CAD build for the part. Positions are in the model's coordinates, mm. A direction names the side the tool comes from. Coordinates: 2 decimals unless noted, no trailing zeros. Write each loop counter-clockwise with the first axis right and the second up, starting at its lowest first coordinate (ties: lowest second). Pieces come first, ordered by that corner, then holes. Notation, with made-up numbers: (-1.5, -24) - (11.5, -24) arc R13 ccw to (11.5, 1) - close; hole circle Ø8 at (52, -38). An arc over 180 degrees is marked (long way). Answer in a Markdown table with one row per item. Add a question column.
Q1. Band-saw the part on D-D (z = 19). List the corners of the cut face in (x, y), and give its area (3 significant figures).
Q2. 3-axis set-ups, long thin cutter, end or side, ignore diameter. For faces 4 (the flat face through (67.5, 25, 17)), 5 (the flat face through (16, 10, 17)), 6 (the flat face through (38, 40, 17)), 7 (the flat face through (72.5, 23, 21)): which of +Z, -Z, +X, -X, +Y, -Y reach the whole face in a straight line?
Q3. Drill centre lines: line 1 along Y through (x, z) = (62, 22); line 2 along X through (y, z) = (21, 26); line 3 along Y through (x, z) = (34.5, 25). Where is each one in solid material? Low to high. Write a range as from..to.
Q4. Band-saw the part on B-B (x = 61). List the corners of the cut face in (y, z).
Q5. Two-plate mould, pull along Y, no slides. Class faces 1 (the flat face through (75, 25, 2)), 2 (the cylindrical face through (1, 48, 3)), 3 (the flat face through (19, 15, 17)): +Y half, -Y half, draft (parallel to the pull), parting line (faces both ways), or undercut.
Q6. Band-saw the part on C-C (y = 25.5). List the corners of the cut face in (x, z), and give its area (3 significant figures).
Q7. Pin check, flat tips, straight feed: pin 1 (1 mm diameter, centred on x = 56, z = 26.5, fed in from -Y); pin 2 (20 mm diameter, centred on x = 29, y = 28, fed in from +Z); pin 3 (7 mm diameter, centred on x = 16, z = 17, fed in from +Y). Stop position of each tip, or through.
Q8. Band-saw the part on A-A (x = 35.5). List the corners of the cut face in (y, z), and give its area (3 significant figures).
```python
from build123d import *

# Parameters (mm, degrees)
F0_W     = 75
F0_H     = 50
F1_DEPTH = 5
F2_R     = 5
F4_DEPTH = 25
F6_DEPTH = 70


with BuildPart() as f1:
    # F0 (on Top) → F1 (new body)
    with BuildSketch(Plane.XY):
        with Locations((37.5, 25)):
            Rectangle(F0_W, F0_H)
    extrude(amount=F1_DEPTH)

    # F2
    f2_edges = [f1.edges().sort_by_distance(p)[0] for p in [
        (75, 0, 2.5),
        (0, 0, 2.5),
        (0, 50, 2.5),
        (75, 50, 2.5),
    ]]
    fillet(f2_edges, radius=F2_R)

    # F3 (on face) → F4 (join)
    with BuildSketch(Plane.XY.offset(5)):
        Polygon((2.5, 40), (2.5, 10), (30, 10), (30, 15), (7.5, 15), (7.5, 35), (67.5, 35), (67.5, 15), (45, 15), (45, 10), (72.5, 10), (72.5, 40), align=None)
    extrude(amount=F4_DEPTH)

    # F5 (on face) → F6 (join)
    with BuildSketch(Plane(origin=(2.5, 0, 0), x_dir=(0, -1, 0), z_dir=(-1, 0, 0))):
        Polygon((-15, 30), (-10, 30), (-4.996269, 46.118304), (-9.996269, 46.118304), align=None)
    extrude(amount=-F6_DEPTH)


solid = f1.part
```
Checked values:
| question | item | result |
|---|---|---|
| 1 | outline | (2.5, 10) - (30, 10) - (30, 15) - (7.5, 15) - (7.5, 35) - (67.5, 35) - (67.5, 15) - (45, 15) - (45, 10) - (72.5, 10) - (72.5, 40) - (2.5, 40) - close |
| 1 | area | 825 mm² |
| 2 | face 4 | +Z |
| 2 | face 5 | +X, -X, -Y |
| 2 | face 6 | +Z, +X, -X, +Y |
| 2 | face 7 | +Z, +X, +Y, -Y |
| 3 | line 1 | y = 10..15, 35..40 |
| 3 | line 2 | x = 2.5..7.5, 67.5..72.5 |
| 3 | line 3 | y = 35..40 |
| 4 | outline | (0, 0) - (50, 0) - (50, 5) - (40, 5) - (40, 30) - (35, 30) - (35, 5) - (15, 5) - (15, 30) - (10, 46.12) - (5, 46.12) - (10, 30) - (10, 5) - (0, 5) - close |
| 5 | face 1 | draft |
| 5 | face 2 | +Y half |
| 5 | face 3 | undercut |
| 6 | outline | (0, 0) - (75, 0) - (75, 5) - (72.5, 5) - (72.5, 30) - (67.5, 30) - (67.5, 5) - (7.5, 5) - (7.5, 30) - (2.5, 30) - (2.5, 5) - (0, 5) - close |
| 6 | area | 625 mm² |
| 7 | pin 1 | stops at y = 10 |
| 7 | pin 2 | stops at z = 30 |
| 7 | pin 3 | stops at y = 40 |
| 8 | outline | (0, 0) - (50, 0) - (50, 5) - (40, 5) - (40, 30) - (35, 30) - (35, 5) - (0, 5) - close; (5, 46.12) - (10, 30) - (15, 30) - (10, 46.12) - close |
| 8 | area | 456 mm² |
